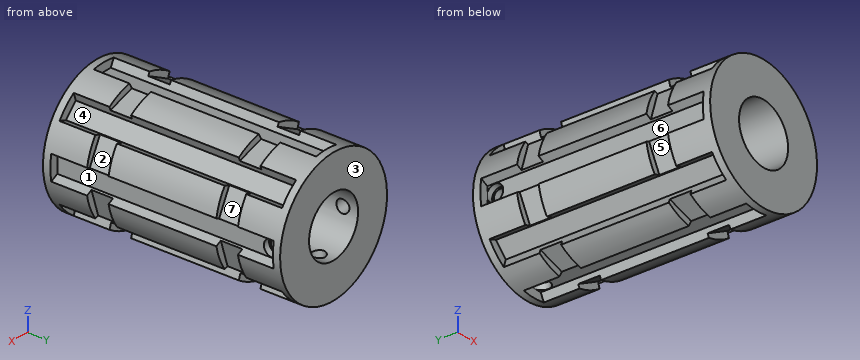
from build123d import *

# Parameters (mm, degrees)
SKETCH1_R           = 15.2785
BOSS_EXTRUDE1_DEPTH = 55
CUT_EXTRUDE2_DEPTH  = 25.8
CIRPATTERN1_COUNT   = 8
SKETCH5_R           = 7.005
CUT_EXTRUDE3_DEPTH  = 60.092005589
SKETCH7_W           = 5
SKETCH7_H           = 1.5
CUT_EXTRUDE4_DEPTH  = 60.092005589
CIRPATTERN2_COUNT   = 8
SKETCH8_R           = 1.9
CUT_EXTRUDE5_DEPTH  = 1.5
CIRPATTERN3_COUNT   = 2
SKETCH9_R           = 1.9
CUT_EXTRUDE6_DEPTH  = 1.5
SKETCH10_R          = 1.505
CUT_EXTRUDE7_DEPTH  = 64.17051378
SKETCH11_R          = 1.505
CUT_EXTRUDE8_DEPTH  = 8


with BuildPart() as part:
    # Sketch1 → Boss-Extrude1 (new body)
    with BuildSketch(Plane(origin=(0, 0, 0), x_dir=(1, 0, 0), z_dir=(0, 1, 0))):
        with Locations(Location((0, 0, 0), (0, 0, 270))):
            Circle(SKETCH1_R)
        with BuildLine():
            Line((1.91637679, 2.5), (-1.91637679, 2.5))
            ThreePointArc((-1.91637679, 2.5), (0, -3.15), (1.91637679, 2.5))
        make_face(mode=Mode.SUBTRACT)
    extrude(amount=BOSS_EXTRUDE1_DEPTH)

    # Sketch3 → Cut-Extrude2 (cut, symmetric)
    with BuildSketch(Plane(origin=(0, 27.5, 0), x_dir=(-1, 0, 0), z_dir=(0, -1, 0))):
        Polygon((-2, 13.2785), (2, 13.2785), (3, 15.2785), (-3, 15.2785), align=None)
    cut_extrude2 = extrude(amount=CUT_EXTRUDE2_DEPTH, both=True, mode=Mode.SUBTRACT)

    # CirPattern1: Cut-Extrude2 ×8 about axis
    cirpattern1_axis = Axis((0, 0, 0), (0, 1, 0))
    for i in range(1, CIRPATTERN1_COUNT):
        add(cut_extrude2.rotate(cirpattern1_axis, i * 360 / CIRPATTERN1_COUNT), mode=Mode.SUBTRACT)

    # Sketch5 → Cut-Extrude3 (cut, through all)
    with BuildSketch(Plane(origin=(0, 55, 0), x_dir=(1, 0, 0), z_dir=(0, 1, 0))):
        with Locations(Location((0, 0, 0), (0, 0, 270))):
            Circle(SKETCH5_R)
    extrude(amount=-CUT_EXTRUDE3_DEPTH, mode=Mode.SUBTRACT)

    # Sketch7 → Cut-Extrude4 (cut, symmetric)
    with BuildSketch(Plane(origin=(0, 0, 0), x_dir=(0, -1, 0), z_dir=(0.8870108331782212, 0, 0.46174861323503485))):
        with Locations((-12.5, 14.5285)):
            Rectangle(SKETCH7_W, SKETCH7_H)
        with Locations((-42.5, 14.5285)):
            Rectangle(SKETCH7_W, SKETCH7_H)
    cut_extrude4 = extrude(amount=CUT_EXTRUDE4_DEPTH, both=True, mode=Mode.SUBTRACT)

    # CirPattern2: Cut-Extrude4 ×8 about axis
    cirpattern2_axis = Axis((0, 0, 0), (0, 1, 0))
    for i in range(1, CIRPATTERN2_COUNT):
        add(cut_extrude4.rotate(cirpattern2_axis, i * 360 / CIRPATTERN2_COUNT), mode=Mode.SUBTRACT)

    # Sketch8 → Cut-Extrude5 (cut)
    with BuildSketch(Plane(origin=(13.2785, 0, 0), x_dir=(0, 0, -1), z_dir=(1, 0, 0))):
        with Locations((0, 51.5)):
            Circle(SKETCH8_R)
    cut_extrude5 = extrude(amount=-CUT_EXTRUDE5_DEPTH, mode=Mode.SUBTRACT)

    # CirPattern3: Cut-Extrude5 ×2 about axis
    cirpattern3_axis = Axis((0, 119.409259796, 0), (0, -1, 0))
    for i in range(1, CIRPATTERN3_COUNT):
        add(cut_extrude5.rotate(cirpattern3_axis, i * 360 / CIRPATTERN3_COUNT), mode=Mode.SUBTRACT)

    # Sketch9 → Cut-Extrude6 (cut)
    with BuildSketch(Plane(origin=(0, 0, -13.2785), x_dir=(-1, 0, 0), z_dir=(0, 0, -1))):
        with Locations((0, 51.5)):
            Circle(SKETCH9_R)
    extrude(amount=-CUT_EXTRUDE6_DEPTH, mode=Mode.SUBTRACT)

    # Sketch10 → Cut-Extrude7 (cut, through all)
    with BuildSketch(Plane(origin=(11.7785, 0, 0), x_dir=(0, 0, -1), z_dir=(1, 0, 0))):
        with Locations((0, 51.5)):
            Circle(SKETCH10_R)
    extrude(amount=-CUT_EXTRUDE7_DEPTH, mode=Mode.SUBTRACT)

    # Sketch11 → Cut-Extrude8 (cut)
    with BuildSketch(Plane(origin=(0, 0, -11.7785), x_dir=(-1, 0, 0), z_dir=(0, 0, -1))):
        with Locations((0, 51.5)):
            Circle(SKETCH11_R)
    extrude(amount=-CUT_EXTRUDE8_DEPTH, mode=Mode.SUBTRACT)


solid = part.part
Here's how the part is built. I have some questions about the finished solid (model axes, mm). Face numbers are marked on the shaded views. A direction names the side the tool comes from. Coordinates: 2 decimals unless noted, no trailing zeros. Write each loop counter-clockwise with the first axis right and the second up, starting at its lowest first coordinate (ties: lowest second). Pieces come first, ordered by that corner, then holes.
Item 1: I want a section at A-A on z = 0. Count the separate pieces of the cut face and the enclosed holes in it, and give its area (3 significant figures).
Item 2: I want a section at D-D on z = 6. Write out the boundary of the cut face in (x, y), and give its area (3 significant figures).
Item 3: Will these pins go through, and if not, where does the flat tip stop? pin 1 (3.5 mm diameter, centred on x = 13.5, z = -5.5, fed in from -Y); pin 2 (3 mm diameter, centred on x = 7.5, y = 8.5, fed in from -Z); pin 3 (2 mm diameter, centred on y = 34.5, z = -0.5, fed in from -X); pin 4 (10 mm diameter, centred on x = 10.5, y = 35.5, fed in from +Z).
Item 4: If I drill on line 1 (X direction, y = 51.5, z = -10.8) (3 decimals); line 2 (Z direction, x = -1.5, y = 23); line 3 (X direction, y = 26, z = 0) (1 decimal), over which ranges is the centre line in solid material (lowest first)?
Item 5: If we mould it in two halves opening along Z, with no side actions, what happens to the marked faces 1, 2 and 3? For each: +Z half, -Z half, draft (parallel to the pull), parting line (faces both ways), or undercut.
Item 6: On a 3-axis mill with a long thin cutter (end or side, diameter ignored), from which of +Z, -Z, +X, -X, +Y, -Y can I reach the whole of each face in a straight line? I mean the marked faces 4, 5, 6 and 7. Say none if no direction works.
Findings below:
1. separate pieces: 4
1. enclosed holes: 0
1. area: 664 mm2
2. outline: (-14.05, 0) - (-3.62, 0) - (-3.62, 55) - (-14.05, 55) - (-14.05, 45) - (-12.56, 45) - (-12.56, 40) - (-14.05, 40) - (-14.05, 15) - (-12.56, 15) - (-12.56, 10) - (-14.05, 10) - close; (3.62, 0) - (14.05, 0) - (14.05, 10) - (12.41, 10) - (12.41, 15) - (14.05, 15) - (14.05, 40) - (12.41, 40) - (12.41, 45) - (14.05, 45) - (14.05, 55) - (3.62, 55) - close
2. area: 1,120 mm2
3. pin 1: stops at y = 0
3. pin 2: stops at z = -14.05
3. pin 3: stops at x = -13.28
3. pin 4: stops at z = 14.25
4. line 1: x = -7.979 to -1.505, 1.505 to 7.979
4. line 2: z = -13.28 to -6.84, 6.84 to 13.28
4. line 3: x = -13.3 to -7, 7 to 13.3
5. face 1: undercut
5. face 2: +Z half
5. face 3: draft
6. face 4: none
6. face 5: -Z, -X
6. face 6: -X
6. face 7: +Z, +X
